Autodesk Inventor part; units mm, degrees
sketch "Sketch1" plane through (0, 0, 0) normal (0, 0, 1) x (1, 0, 0)
  line L0 (-25, 25) -> (25, 25)
  line L1 (25, 25) -> (25, -25)
  line L2 (25, -25) -> (-25, -25)
  line L3 (-25, -25) -> (-25, 25)
  line L4 (-25, 25) -> (25, -25) construction
  line L5 (25, 25) -> (-25, -25) construction
  line L6 (-22, 22) -> (22, 22)
  line L7 (22, 22) -> (22, -22)
  line L8 (22, -22) -> (-22, -22)
  line L9 (-22, -22) -> (-22, 22)
  line L10 (-22, 22) -> (22, -22) construction
  line L11 (22, 22) -> (-22, -22) construction
  point P0 (0, 0)
  point P1 (0, 0)
  dimension "d0" = 50
  dimension "d1" = 3
extrude "Extrusion1" add sketch "Sketch1" along normal mid plane 730
properties part number "perna" material "Wood (Walnut)"
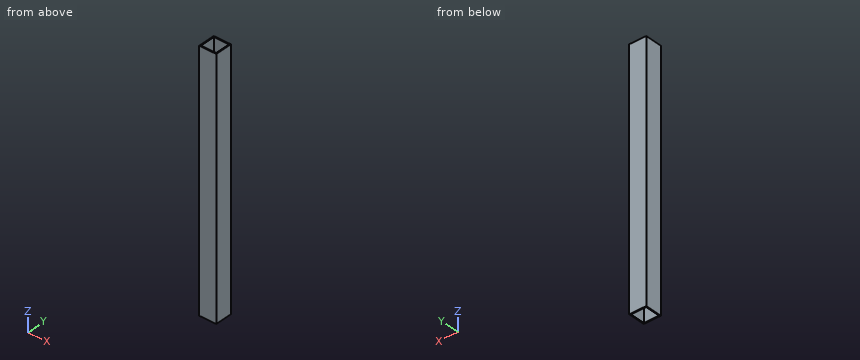
The model under review builds one solid part; all positions refer to its coordinate system, in mm. Coordinates: 2 decimals unless noted, no trailing zeros. Order: outer loops, then holes, each group sorted by start corner. A loop starts at its lowest first (then second) coordinate and runs counter-clockwise, first axis right, second up. Notation, with made-up numbers: (-13.75, 35.5) -> (31.25, 35.5) arc R11 cw to (31.25, 44.5) -> close; hole circle Ø8 at (67.25, 63.25). An arc over 180 degrees is marked (long way). Answer in a Markdown table with one row per item. Add a question column.
Item 1: We need section A-A on x = 10. Write out the cut boundary in (y, z), plus the area to 3 significant figures.
Item 2: We need section C-C on z = -66.5. Write out the cut boundary in (x, y).
Item 3: To check wall thickness, follow probe 1 along Y at (x, z) = (17, -317). State the ranges of the line that lie inside material, in increasing order.
Final values:
| question | item | result |
|---|---|---|
| 1 | outline | (-25, -365) -> (-22, -365) -> (-22, 365) -> (-25, 365) -> close; (22, -365) -> (25, -365) -> (25, 365) -> (22, 365) -> close |
| 1 | area | 4,380 mm2 |
| 2 | outline | (-25, -25) -> (25, -25) -> (25, 25) -> (-25, 25) -> close; hole (-22, -22) -> (22, -22) -> (22, 22) -> (-22, 22) -> close |
| 3 | probe 1 | y = -25 to -22, 22 to 25 |
